Could you check a few things on this model? Use its own coordinates, in mm. Face numbers are marked on the shaded views. A direction names the side the tool comes from. Round coordinates to 2 decimals unless told otherwise and drop trailing zeros. Write each loop counter-clockwise with the first axis right and the second up, starting at its lowest first coordinate (ties: lowest second). Pieces come first, ordered by that corner, then holes. Notation, with made-up numbers: M -30.5,36 L 18.5,36 A35 ccw 18.5,71 Z; hole C -12,3 d7. An arc over 180 degrees is marked long. One line per item, written item: value. Start each with the question number.
(1) If I drill on L1, parallel to Z at x = -0.9, y = 0 (3 decimals); L2, parallel to Y at x = 0.8, z = 30 (3 decimals); L3, parallel to X at y = 1.25, z = 13.5, over which ranges is the centre line in solid material (lowest first)?
(2) I want a section at D-D on z = 11. Please give me the cut outline in (x, y).
(3) Which directions (+Z, -Z, +X, -X, +Y, -Y) give clear straight access to the entire face, cutting with the end or side of a thin tool? Please do the marked faces 1, 2, 3, 4 and 5.
(4) I want a section at B-B on y = 0. Please give me the cut outline in (x, z) (3 decimals), and give its area (3 significant figures).
(5) I'm going to push flat-ended pins straight in: pin 1 Ø2.5 at (y, z) = (-1, 5) entering from +X; pin 2 Ø0.5 at (x, z) = (0, -0.5) entering from -Y (3 decimals); pin 3 Ø1.5 at (x, z) = (-0.5, 10.5) entering from -Y; pin 4 Ø2 at (x, y) = (-3, -2) entering from +Z. Where does each tip first touch, or does it pass through?
(6) I want a section at A-A on z = 30. Please give me the cut outline in (x, y) (3 decimals), and give its area (3 significant figures).
(7) I want a section at C-C on x = 0.5. Please give me the cut outline in (y, z) (3 decimals), and give its area (3 significant figures).
Autodesk Inventor part; units mm, degrees
ref_plane "YZ Plane" through (0, 0, 0) normal (1, 0, 0) x (0, 1, 0)
ref_plane "XZ Plane" through (0, 0, 0) normal (0, 1, 0) x (-1, 0, 0)
ref_plane "XY Plane" through (0, 0, 0) normal (0, 0, 1) x (1, 0, 0)
sketch "Sketch1" plane through (0, 0, 0) normal (0, 0, 1) x (1, 0, 0)
  line L0 (-3.175, -3.175) -> (-3.175, 3.175)
  line L1 (-3.175, 3.175) -> (3.175, 3.175)
  line L2 (3.175, 3.175) -> (3.175, -3.175)
  line L3 (3.175, -3.175) -> (-3.175, -3.175)
  line L4 (-5, -5) -> (5, -5)
  line L5 (5, -5) -> (5, 5)
  line L6 (5, 5) -> (-5, 5)
  line L7 (-5, 5) -> (-5, -5)
  line L8 (-4.1303, 4.1303) -> (4.1303, 4.1303)
  line L9 (4.1303, 4.1303) -> (4.1303, -4.1303)
  line L10 (-4.1303, -4.1303) -> (-4.1303, 4.1303)
  line L11 (4.1303, -4.1303) -> (-4.1303, -4.1303)
  line L12 (2.54, -2.54) -> (-2.54, -2.54)
  line L13 (-2.54, -2.54) -> (-2.54, 2.54)
  line L14 (-2.54, 2.54) -> (2.54, 2.54)
  line L15 (2.54, 2.54) -> (2.54, -2.54)
  line L16 (2.54, -2.54) -> (-2.54, 2.54) construction
  line L17 (-2.54, -2.54) -> (2.54, 2.54) construction
  point P0 (0, 0)
  dimension "d0" = 5.08
  dimension "d1" = 5.08
extrude "Extrusion1" add sketch "Sketch1" along normal blind 25 contours L12 L13 L14 L15
sketch "Sketch2" plane through (0, 0, 0) normal (0, 0, -1) x (-1, 0, 0)
  line L0 (-3.175, -3.175) -> (-3.175, 3.175)
  line L1 (3.175, 3.175) -> (3.175, -3.175)
  line L2 (-3.175, -3.175) -> (3.175, -3.175)
  line L3 (3.175, -3.175) -> (3.175, 3.175)
  line L4 (3.175, 3.175) -> (-3.175, 3.175)
  line L5 (-3.175, 3.175) -> (-3.175, -3.175)
  point P0 (0, 0)
extrude "Extrusion2" add sketch "Sketch2" along normal blind 1
sketch "Sketch3" plane through (0, 0, 25) normal (0, 0, 1) x (1, 0, 0)
  line L0 (3.75, -4) -> (-3.75, -4)
  line L1 (-3.75, -4) -> (-3.75, 4)
  line L2 (-3.75, 4) -> (3.75, 4)
  line L3 (3.75, 4) -> (3.75, -4)
  line L4 (3.75, -4) -> (-3.75, 4) construction
  line L5 (-3.75, -4) -> (3.75, 4) construction
  point P0 (0, 0)
  dimension "d6" = 7.5
  dimension "d7" = 8
extrude "Extrusion3" add sketch "Sketch3" along normal blind 1 and the other way blind 2
fillet "Fillet1" radius 5 4 edges at (0, 2.54, 23) (2.54, 0, 23) (-2.54, 0, 23) (0, -2.54, 23)
sketch "Sketch4" plane through (0, 0, 26) normal (0, 0, 1) x (1, 0, 0)
  line L0 (2.5088, -3.4457) -> (-2.5088, -3.4457)
  line L1 (-2.5088, -3.4457) -> (-2.5088, 3.4457)
  line L2 (-2.5088, 3.4457) -> (2.5088, 3.4457)
  line L3 (2.5088, 3.4457) -> (2.5088, -3.4457)
  line L4 (2.5088, -3.4457) -> (-2.5088, 3.4457) construction
  line L5 (-2.5088, -3.4457) -> (2.5088, 3.4457) construction
  point P0 (0, 0)
extrude "Extrusion4" add sketch "Sketch4" along normal blind 7
sketch "Sketch5" plane through (-2.5088, -3.4457, 26) normal (-1, 0, 0) x (0, 0, 1)
  line L0 (0, 6.8913) -> (7, 6.8913)
  line L1 (0, 0) -> (4, 0)
  line L2 (4, 0) -> (4, 6.8913)
  line L3 (4, 6.8913) -> (0, 6.8913)
  line L4 (0, 6.8913) -> (0, 0)
  circle A0 centre (4, 3.4457) radius 2.125
  point P0 (-26, 3.4457)
  dimension "d15" = 4
  dimension "d16" = 4.25
extrude "Extrusion5" cut sketch "Sketch5" against normal blind 7 contours A0 L2 | L2 A0
fillet "Fillet2" radius 1 4 edges at (-2.5088, 0, 26) (0, -3.4457, 26) (2.5088, 0, 26) (0, 3.4457, 26)
fillet "Fillet3" radius 2 2 edges at (0, -3.4457, 33) (0, 3.4457, 33)
properties part number "arm-seg2"
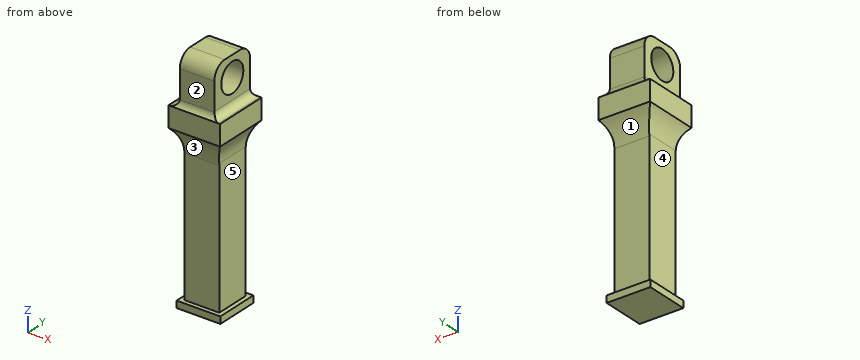
Found:
1. L1: z = -1 to 27.875, 32.125 to 33
1. L2: y = -3.446 to -2.125, 2.125 to 3.446
1. L3: x = -2.54 to 2.54
2. outline: M -2.54,-2.54 L 2.54,-2.54 L 2.54,2.54 L -2.54,2.54 Z
3. face 1: +X, -X, +Y
3. face 2: +Z, +X, -X, -Y
3. face 3: +X, -X, -Y
3. face 4: -X, +Y, -Y
3. face 5: +X, +Y, -Y
4. outline: M -3.75,23 A5 cw -2.54,19.739 L -2.54,0 L -3.175,0 L -3.175,-1 L 3.175,-1 L 3.175,0 L 2.54,0 L 2.54,19.739 A5 cw 3.75,23 L 3.75,26 L 3.509,26 A1 cw 2.509,27 L 2.509,27.875 L -2.509,27.875 L -2.509,27 A1 cw -3.509,26 L -3.75,26 Z; M -2.509,32.125 L 2.509,32.125 L 2.509,33 L -2.509,33 Z
4. area: 162 mm²
5. pin 1: stops at x = 2.54
5. pin 2: stops at y = -3.175
5. pin 3: stops at y = -2.54
5. pin 4: stops at z = 33
6. outline: M -2.509,-3.446 L 2.509,-3.446 L 2.509,-2.125 L -2.509,-2.125 Z; M -2.509,2.125 L 2.509,2.125 L 2.509,3.446 L -2.509,3.446 Z
6. area: 13.3 mm²
7. outline: M -4,23 A5 cw -2.54,19.469 L -2.54,0 L -3.175,0 L -3.175,-1 L 3.175,-1 L 3.175,0 L 2.54,0 L 2.54,19.469 A5 cw 4,23 L 4,26 A1 cw 3.446,26.895 L 3.446,31 A2 ccw 1.446,33 L -1.446,33 A2 ccw -3.446,31 L -3.446,26.895 A1 cw -4,26 Z; hole C 0,30 d4.25
7. area: 183 mm²
